from build123d import *

# Parameters (mm, degrees)
SKETCH1_R           = 1
SKETCH1_R_2         = 4
BOSS_EXTRUDE1_DEPTH = 3
BOSS_EXTRUDE2_START = -10
BOSS_EXTRUDE2_DEPTH = 10
SKETCH2_R           = 1.75
CUT_EXTRUDE1_DEPTH  = 2
FILLET1_DEPTH       = 4
FILLET1_START       = -10
FILLET1_2_DEPTH     = 10


with BuildPart() as part:
    # Sketch1 → Boss-Extrude1 (new body)
    with BuildSketch(Plane(origin=(0, 0, 0), x_dir=(1, 0, 0), z_dir=(0, 1, 0))):
        with BuildLine():
            ThreePointArc((18.051481703, -14.829547427), (41.662522, -8.486422092), (65.646603069, -13.227763489))
            add(Edge.make_bspline(
                [(65.646603069, -13.227763489), (56.529791546, -4.297397801), (30.90013189, 4.342634152), (1.753021735, 9.641935221)],
                knots=[0.6061191, 0.6061191, 0.6061191, 0.6061191, 1.438179848, 1.438179848, 1.438179848, 1.438179848], degree=3))
            ThreePointArc((1.753021735, 9.641935221), (-9.569441867, 2.113239778), (-2.470487043, -9.483495862))
            Line((-2.470487043, -9.483495862), (18.051481703, -14.829547427))
        make_face()
        with Locations(Location((0, 7.05, 0), (0, 0, 270))):
            Circle(SKETCH1_R, mode=Mode.SUBTRACT)
        with Locations(Location((0, -7.05, 0), (0, 0, 270))):
            Circle(SKETCH1_R, mode=Mode.SUBTRACT)
        with Locations(Location((-4.985102807, -4.985102807, 0), (0, 0, 270))):
            Circle(SKETCH1_R, mode=Mode.SUBTRACT)
        with Locations(Location((4.985102807, -4.985102807, 0), (0, 0, 270))):
            Circle(SKETCH1_R, mode=Mode.SUBTRACT)
        with Locations(Location((-7.05, 0, 0), (0, 0, 270))):
            Circle(SKETCH1_R, mode=Mode.SUBTRACT)
        with Locations(Location((0, 0, 0), (0, 0, 270))):
            Circle(SKETCH1_R_2, mode=Mode.SUBTRACT)
        with Locations(Location((7.05, 0, 0), (0, 0, 270))):
            Circle(SKETCH1_R, mode=Mode.SUBTRACT)
        with Locations(Location((-4.985102807, 4.985102807, 0), (0, 0, 270))):
            Circle(SKETCH1_R, mode=Mode.SUBTRACT)
        with Locations(Location((4.985102807, 4.985102807, 0), (0, 0, 270))):
            Circle(SKETCH1_R, mode=Mode.SUBTRACT)
    extrude(amount=BOSS_EXTRUDE1_DEPTH)

    # Sketch1<3> → Boss-Extrude2 (add)
    with BuildSketch(Plane(origin=(0, 0, 0), x_dir=(1, 0, 0), z_dir=(0, 1, 0)).offset(BOSS_EXTRUDE2_START)):
        with BuildLine():
            Line((18.051481703, -14.829547427), (22.89, -16.09))
            ThreePointArc((22.89, -16.09), (46.274614562, -11.793991127), (69.041958929, -18.64555452))
            add(Edge.make_bspline(
                [(65.646603069, -13.227763489), (67.486697691, -15.030226755), (68.654100184, -16.844517492), (69.041958929, -18.64555452)],
                knots=[0.832060748, 0.832060748, 0.832060748, 0.832060748, 1, 1, 1, 1], degree=3))
            ThreePointArc((65.646603069, -13.227763489), (41.662522, -8.486422092), (18.051481703, -14.829547427))
        make_face()
        with BuildLine():
            Line((13.212963406, -13.569094854), (18.051481703, -14.829547427))
            ThreePointArc((18.051481703, -14.829547427), (41.662522, -8.486422092), (65.646603069, -13.227763489))
            add(Edge.make_bspline(
                [(54.827143585, -6.078086241), (59.477760605, -8.399185567), (63.170981642, -10.802770431), (65.646603069, -13.227763489)],
                knots=[0.6061191, 0.6061191, 0.6061191, 0.6061191, 0.832060748, 0.832060748, 0.832060748, 0.832060748], degree=3))
            ThreePointArc((54.827143585, -6.078086241), (33.305217678, -5.852522289), (13.212963406, -13.569094854))
        make_face()
    extrude(amount=BOSS_EXTRUDE2_DEPTH)

    # Sketch2 → Cut-Extrude1 (cut)
    with BuildSketch(Plane(origin=(0, 3, 0), x_dir=(1, 0, 0), z_dir=(0, 1, 0))):
        with Locations(Location((0, 7.05, 0), (0, 0, 270))):
            Circle(SKETCH2_R)
        with Locations(Location((4.985102807, 4.985102807, 0), (0, 0, 270))):
            Circle(SKETCH2_R)
        with Locations(Location((7.05, 0, 0), (0, 0, 270))):
            Circle(SKETCH2_R)
        with Locations(Location((4.985102807, -4.985102807, 0), (0, 0, 270))):
            Circle(SKETCH2_R)
        with Locations(Location((0, -7.05, 0), (0, 0, 270))):
            Circle(SKETCH2_R)
        with Locations(Location((-4.985102807, -4.985102807, 0), (0, 0, 270))):
            Circle(SKETCH2_R)
        with Locations(Location((-7.05, 0, 0), (0, 0, 270))):
            Circle(SKETCH2_R)
        with Locations(Location((-4.985102807, 4.985102807, 0), (0, 0, 270))):
            Circle(SKETCH2_R)
    extrude(amount=-CUT_EXTRUDE1_DEPTH, mode=Mode.SUBTRACT)

    # Fillet1: read off the stored shape, not the designer's step
    # Fillet1 outline → Fillet1 (cut)
    with BuildSketch(Plane(origin=(0, 0, 0), x_dir=(1, 0, 0), z_dir=(0, 1, 0))):
        with BuildLine():
            add(Edge.make_bspline(
                [(56.770531977, -7.082884332), (60.513292136, -9.089900017), (63.526462064, -11.150981005), (65.646603069, -13.227763489)],
                knots=[0.638562604, 0.638562604, 0.638562604, 0.638562604, 0.832060748, 0.832060748, 0.832060748, 0.832060748], degree=3))
            ThreePointArc((56.770531977, -7.082884332), (57.465125309, -8.934236095), (55.720831584, -9.865580632))
            ThreePointArc((55.720831584, -9.865580632), (60.765635031, -11.304836191), (65.646603069, -13.227763489))
        make_face()
        with BuildLine():
            ThreePointArc((18.559470243, -14.56123833), (18.034960356, -14.721619309), (17.487859224, -14.682721609))
            Line((17.487859224, -14.682721609), (18.051481703, -14.829547427))
            ThreePointArc((18.051481703, -14.829547427), (18.305118454, -14.69471599), (18.559470243, -14.56123833))
        make_face()
    extrude(amount=FILLET1_DEPTH, mode=Mode.SUBTRACT)

    # Fillet1 2 outline → Fillet1 2 (cut)
    with BuildSketch(Plane(origin=(0, 0, 0), x_dir=(1, 0, 0), z_dir=(0, 1, 0)).offset(FILLET1_START)):
        with BuildLine():
            ThreePointArc((54.827143585, -6.078086241), (54.727119613, -6.058000301), (54.627060101, -6.038092157))
            ThreePointArc((54.627060101, -6.038092157), (54.822409803, -6.090686613), (55.008905492, -6.169089678))
            add(Edge.make_bspline(
                [(54.827143585, -6.078086241), (54.887894452, -6.10840669), (54.948481948, -6.138741214), (55.008905492, -6.169089678)],
                knots=[0.6061191, 0.6061191, 0.6061191, 0.6061191, 0.609070569, 0.609070569, 0.609070569, 0.609070569], degree=3))
        make_face()
        with BuildLine():
            ThreePointArc((16.754219894, -14.49160575), (15.642770878, -13.216507508), (16.425540404, -11.717018824))
            ThreePointArc((16.425540404, -11.717018824), (14.804293031, -12.617109451), (13.212963406, -13.569094854))
            Line((13.212963406, -13.569094854), (16.754219894, -14.49160575))
        make_face()
    extrude(amount=FILLET1_2_DEPTH, mode=Mode.SUBTRACT)


solid = part.part
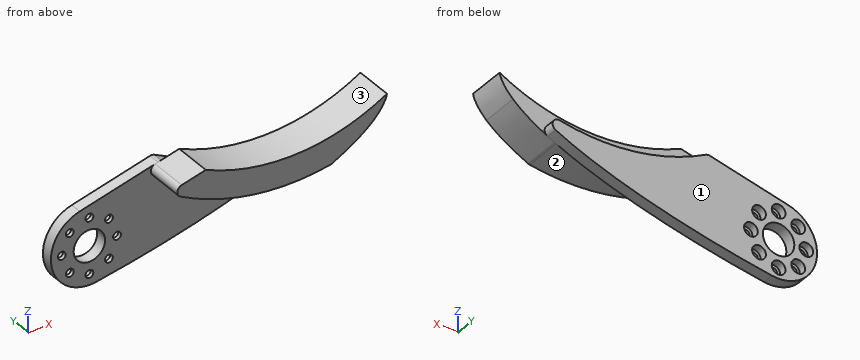
CAD build for the part. Positions are in the model's coordinates, mm. Face numbers are marked on the shaded views. Coordinates: 2 decimals unless noted, no trailing zeros. Order: outer loops, then holes, each group sorted by start corner. A loop starts at its lowest first (then second) coordinate and runs counter-clockwise, first axis right, second up.
Item 1: Band-saw the part on B-B on y = 2. Give the number of separate pieces and of enclosed holes in the cut face, plus the area to 3 significant figures.
Check sheet entries:
separate pieces: 1
enclosed holes: 9
area: 803 mm2
Item 2: Band-saw the part on A-A on x = 0. List the corners of the cut face in (y, z), plus the area to 3 significant figures.
Check sheet entries:
outline: (0, -9.8) - (3, -9.8) - (3, -8.8) - (1, -8.8) - (1, -8.05) - (0, -8.05) - close; (0, -6.05) - (1, -6.05) - (1, -5.3) - (3, -5.3) - (3, -4) - (0, -4) - close; (0, 4) - (3, 4) - (3, 5.3) - (1, 5.3) - (1, 6.05) - (0, 6.05) - close; (0, 8.05) - (1, 8.05) - (1, 8.8) - (3, 8.8) - (3, 10.13) - (0, 10.13) - close
area: 17.8 mm2
Item 3: Two-plate mould, pull along X, no slides. Class the marked faces 1, 2 and 3: +X half, -X half, draft (parallel to the pull), parting line (faces both ways), or undercut.
Check sheet entries:
face 1: draft
face 2: parting line
face 3: undercut
Item 4: Drill centre lines: L1, parallel to Y at x = 11, z = -6.75; L2, parallel to Y at x = 65, z = 15.25; L3, parallel to X at y = 1.5, z = 7.05. Where is each one in solid material? Low to high.
Check sheet entries:
L1: y = 0 to 3
L2: y = -10 to 0
L3: x = -6.81 to -1.75, 1.75 to 56.71
Item 5: Pin check, flat tips, straight feed: pin 1 Ø1.8 at (x, z) = (-5.5, 5) entering from +Y; pin 2 Ø2 at (y, z) = (-3, 11) entering from +X; pin 3 Ø4 at (x, z) = (-4.99, -4.99) entering from -Y. Stop position of each tip, or through.
Check sheet entries:
pin 1: stops at y = 1
pin 2: stops at x = 64.29
pin 3: stops at y = 0
